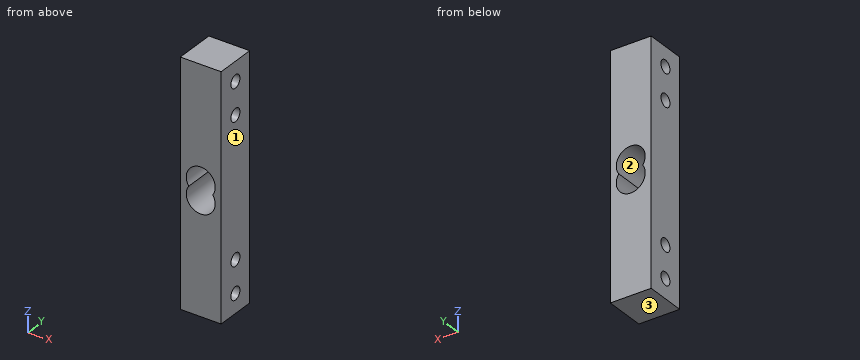
```python
from build123d import *

# Parameters (mm, degrees)
SKETCH1_W           = 12.7
SKETCH1_H           = 12.7
BOSS_EXTRUDE1_DEPTH = 37.5
SKETCH2_R           = 2
CUT_EXTRUDE1_DEPTH  = 80
CUT_EXTRUDE2_DEPTH  = 80


with BuildPart() as part:
    # Sketch1 → Boss-Extrude1 (new, symmetric)
    with BuildSketch(Plane.XY):
        Rectangle(SKETCH1_W, SKETCH1_H)
    extrude(amount=BOSS_EXTRUDE1_DEPTH, both=True)

    # Sketch2 → Cut-Extrude1 (cut)
    with BuildSketch(Plane(origin=(6.35, 0, 0), x_dir=(0, 0, -1), z_dir=(1, 0, 0))):
        with Locations((-31.5, 0)):
            Circle(SKETCH2_R)
        with Locations((-21.5, 0)):
            Circle(SKETCH2_R)
        with Locations((21.5, 0)):
            Circle(SKETCH2_R)
        with Locations((31.5, 0)):
            Circle(SKETCH2_R)
    extrude(amount=-CUT_EXTRUDE1_DEPTH, mode=Mode.SUBTRACT)

    # Sketch3 → Cut-Extrude2 (cut)
    with BuildSketch(Plane.XZ.offset(6.35)):
        with BuildLine():
            ThreePointArc((3.741657387, 0), (0, 7), (-3.741657387, 0))
            ThreePointArc((-3.741657387, 0), (0, -7), (3.741657387, 0))
        make_face()
    extrude(amount=-CUT_EXTRUDE2_DEPTH, mode=Mode.SUBTRACT)


solid = part.part
```
Geometry: final body of the model. Coordinates: model frame, mm. Face numbers are marked on the shaded views. Round coordinates to 2 decimals unless told otherwise and drop trailing zeros. Write each loop counter-clockwise with the first axis right and the second up, starting at its lowest first coordinate (ties: lowest second). Pieces come first, ordered by that corner, then holes.
Item 1: Material intervals for L1, parallel to Y at x = 0.5, z = 31.5; L2, parallel to Z at x = -2.5, y = -1.5; L3, parallel to X at y = -2.75, z = 2.5, sorted ascending.
Item 2: Section query B-B (z = 21.5). Return loops of the section in (x, y), plus the area to 3 significant figures.
Item 3: Section query D-D (z = -2.5). Return loops of the section in (x, y), plus the area to 3 significant figures.
Item 4: Section query C-C (y = -0.75). Return loops of the section in (x, z), plus the area to 3 significant figures.
Item 5: Section query A-A (x = 0). Return loops of the section in (y, z), plus the area to 3 significant figures.
Item 6: Mould query, pull axis X, two halves, no side actions, for the marked faces 1, 2 and 3. Classes: +X half, -X half, draft (parallel to the pull), parting line (faces both ways), or undercut.
Completed:
1. L1: y = -6.35 to -2, 2 to 6.35
1. L2: z = -37.5 to -32.82, -30.18 to -22.82, -20.18 to -6.24, 6.24 to 20.18, 22.82 to 30.18, 32.82 to 37.5
1. L3: x = -6.35 to -4.5, 4.5 to 6.35
2. outline: (-6.35, -6.35) - (6.35, -6.35) - (6.35, -2) - (-6.35, -2) - close; (-6.35, 2) - (6.35, 2) - (6.35, 6.35) - (-6.35, 6.35) - close
2. area: 110 mm2
3. outline: (-6.35, -6.35) - (-4.5, -6.35) - (-4.5, 6.35) - (-6.35, 6.35) - close; (4.5, -6.35) - (6.35, -6.35) - (6.35, 6.35) - (4.5, 6.35) - close
3. area: 47.0 mm2
4. outline: (-6.35, -37.5) - (6.35, -37.5) - (6.35, -33.35) - (-6.35, -33.35) - close; (-6.35, -29.65) - (6.35, -29.65) - (6.35, -23.35) - (-6.35, -23.35) - close; (-6.35, -19.65) - (6.35, -19.65) - (6.35, 19.65) - (-6.35, 19.65) - close; (-6.35, 23.35) - (6.35, 23.35) - (6.35, 29.65) - (-6.35, 29.65) - close; (-6.35, 33.35) - (6.35, 33.35) - (6.35, 37.5) - (-6.35, 37.5) - close; hole (-3.74, 0) arc R4.5 ccw (long way) to (3.74, 0) arc R4.5 ccw (long way) to start
4. area: 658 mm2
5. outline: (-6.35, -37.5) - (6.35, -37.5) - (6.35, -7) - (-6.35, -7) - close; (-6.35, 7) - (6.35, 7) - (6.35, 37.5) - (-6.35, 37.5) - close; hole circle Ø4 at (0, -31.5); hole circle Ø4 at (0, -21.5); hole circle Ø4 at (0, 21.5); hole circle Ø4 at (0, 31.5)
5. area: 724 mm2
6. face 1: +X half
6. face 2: undercut
6. face 3: draft
